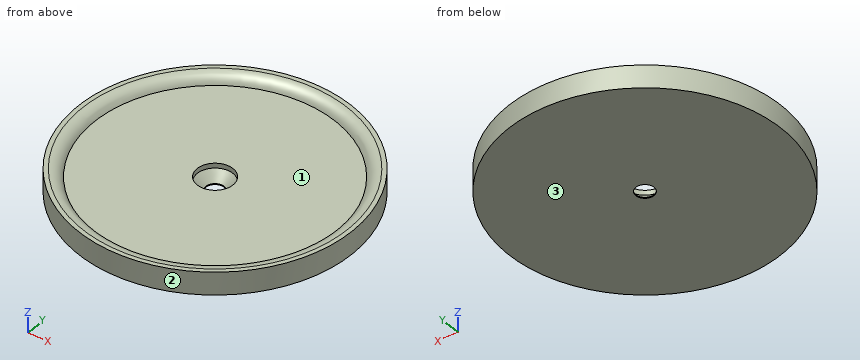
from build123d import *

# Parameters (mm, degrees)
F0_R        = 18.5
F0_R_2      = 1.4
F1_DEPTH    = 2.25
F2_R        = 2.75
F3_DEPTH    = 0.1
F4_S5_R     = 2.75
F4_T6_DEPTH = 6
F6_W        = 2.5
F6_H        = 3.5


# Not quite as in the source:
# - a fillet or chamfer that OpenCascade refuses, or shapes differently, is made with other operations: its cross-section is extruded or revolved along the edge and cut away or added
# - a feature names something its author has since deleted; it is built from what else it names


with BuildPart() as f1:
    # F0 (on Top) → F1 (new body)
    with BuildSketch(Plane.XY):
        Circle(F0_R)
        Circle(F0_R_2, mode=Mode.SUBTRACT)
    extrude(amount=F1_DEPTH)

    # F2 (on face) → F3 (cut)
    with BuildSketch(Plane.XY.offset(2.25)):
        Circle(F2_R)
    extrude(amount=-F3_DEPTH, mode=Mode.SUBTRACT)

    # F4: chamfer of 2 on 1 edges, made by hand


with BuildPart() as f4_tool2:
    # F4_s3 → F4_t4 (revolve)
    with BuildSketch(Plane.XZ):
        Polygon((1.4, 0.15), (3.4, 2.15), (1.4, 2.15), align=None)
    revolve(axis=Axis((0, 0, 2.15), (0, 0, -1)))

    # F4_s5 → F4_t6 (intersect, symmetric)
    with BuildSketch(Plane.XY.offset(1.2)):
        Circle(F4_S5_R)
    extrude(amount=F4_T6_DEPTH, both=True, mode=Mode.INTERSECT)


with BuildPart() as f1_1:
    add(f1.part)

    # F4_t1: cut F4_tool2
    add(f4_tool2.part, mode=Mode.SUBTRACT)

    # F6 (on Right) → F7 (revolve)
    with BuildSketch(Plane.YZ):
        with Locations((-19.75, 1.75)):
            Rectangle(F6_W, F6_H)
    revolve(axis=Axis((0, 0, 7.0907436311), (0, 0, 1)))

    # F8: fillet of radius 2 on 1 edges, made by hand

    # F8_s1 → F8_t2 (revolve, cut)
    with BuildSketch(Plane.YZ):
        with BuildLine():
            ThreePointArc((-20.3540496218, 3.5), (-19.236015633, 3.1583123952), (-18.5, 2.25))
            Line((-18.5, 2.25), (-18.5, 3.5))
            Line((-18.5, 3.5), (-20.3540496218, 3.5))
        make_face()
    revolve(axis=Axis((0, 0, 3.5), (0, 0, 1)), mode=Mode.SUBTRACT)


solid = f1_1.part
The model under review builds one solid part; all positions refer to its coordinate system, in mm. Face numbers are marked on the shaded views. Give positions to 0.01 mm unless a question says otherwise; leave off trailing zeros. Order: outer loops, then holes, each group sorted by start corner. A loop starts at its lowest first (then second) coordinate and runs counter-clockwise, first axis right, second up. Notation, with made-up numbers: M 33,61 L 87,61 A22 ccw 87,69 Z; hole C -23,81.25 d9. An arc over 180 degrees is marked long. Answer in a Markdown table with one row per item. Add a question column.
1. Add section A-A on x = 0. State the section outline as (y, z) points, plus the area to 3 significant figures.
2. Mouldability with a two-part tool opening along X and no side actions: class the marked faces 1, 2 and 3 as released by +X, released by -X, zero draft, split by the parting line, or undercut.
3. For pin 1 Ø2 at (x, z) = (7.5, 1) entering from -Y; pin 2 Ø10 at (x, y) = (10, -10) entering from +Z; pin 3 Ø2 at (x, y) = (0, 0) entering from -Z, all flat-tipped, find the tip position at first contact; note any pin that passes through.
4. Add section C-C on z = 0.9. State the section outline as (x, y) points, plus the area to 3 significant figures.
5. To check wall thickness, follow line 1 along Z through (x, y) = (-14, -9); line 2 along X through (y, z) = (0, 0.1); line 3 along X through (y, z) = (6.5, 2.35). State the ranges of each line that lie inside material, in increasing order.
The answers:
| question | item | result |
|---|---|---|
| 1 | outline | M -21,0 L -1.4,0 L -1.4,0.15 L -2.75,1.5 L -2.75,2.25 L -18.5,2.25 A2 ccw -20.35,3.5 L -21,3.5 Z; M 1.4,0 L 21,0 L 21,3.5 L 20.35,3.5 A2 ccw 18.5,2.25 L 2.75,2.25 L 2.75,1.5 L 1.4,0.15 Z |
| 1 | area | 89.3 mm2 |
| 2 | face 1 | undercut |
| 2 | face 2 | split by the parting line |
| 2 | face 3 | zero draft |
| 3 | pin 1 | y = -19.97 |
| 3 | pin 2 | z = 3.09 |
| 3 | pin 3 | through |
| 4 | outline | C 0,0 d42; hole C 0,0 d4.3 |
| 4 | area | 1,370 mm2 |
| 5 | line 1 | 0 to 2.25 |
| 5 | line 2 | -21 to -1.4, 1.4 to 21 |
| 5 | line 3 | -19.97 to -17.37, 17.37 to 19.97 |
